Verification items for the finished model (mm, model axes). A direction names the side the tool comes from. Give positions to 0.01 mm unless a question says otherwise; leave off trailing zeros. Loops run counter-clockwise (first coordinate to the right, second up) from the corner with the lowest first, then second, coordinate; pieces in that order, holes last. Notation, with made-up numbers: M 39,36 L 43,36 A22 cw 43,60 Z; hole C 82.25,-23 d10. An arc over 180 degrees is marked long. Use CSV: the item, a comma, the result in double quotes.
from build123d import *

# Parameters (mm, degrees)
SKETCH1_R           = 1.905
BOSS_EXTRUDE1_DEPTH = 6.35
BOSS_EXTRUDE2_START = -6.35
BOSS_EXTRUDE2_DEPTH = 6.35
BOSS_EXTRUDE4_START = -6.35
SKETCH6_R           = 1.905
BOSS_EXTRUDE4_DEPTH = 6.35
SKETCH7_R           = 1.905
CUT_EXTRUDE3_DEPTH  = 15.340319034
SKETCH8_R           = 3.048
CUT_EXTRUDE4_DEPTH  = 2.54


with BuildPart() as part:
    # Sketch1 → Boss-Extrude1 (new body)
    with BuildSketch(Plane.YZ):
        with BuildLine():
            Line((-3.175, 0), (-3.175, -7.62))
            ThreePointArc((-3.175, -7.62), (0, -10.795), (3.175, -7.62))
            Line((3.175, -7.62), (3.175, 0))
            ThreePointArc((3.175, 0), (0, 3.175), (-3.175, 0))
        make_face()
        with Locations(Location((0, 0, 0), (0, 0, 270))):
            Circle(SKETCH1_R, mode=Mode.SUBTRACT)
    extrude(amount=BOSS_EXTRUDE1_DEPTH)

    # Sketch2 → Boss-Extrude2 (add)
    with BuildSketch(Plane.YZ.offset(6.35).offset(BOSS_EXTRUDE2_START)):
        with BuildLine():
            Line((4.445, -7.62), (4.445, 0))
            ThreePointArc((4.445, 0), (0, 4.445), (-4.445, 0))
            Line((-4.445, 0), (-4.445, -7.62))
            ThreePointArc((-4.445, -7.62), (0, -12.065), (4.445, -7.62))
        make_face()
        with BuildLine():
            ThreePointArc((3.175, 0), (0, 3.175), (-3.175, 0))
            Line((-3.175, 0), (-3.175, -7.62))
            ThreePointArc((-3.175, -7.62), (0, -10.795), (3.175, -7.62))
            Line((3.175, -7.62), (3.175, 0))
        make_face(mode=Mode.SUBTRACT)
    extrude(amount=BOSS_EXTRUDE2_DEPTH)

    # Sketch6 → Boss-Extrude4 (add)
    with BuildSketch(Plane.YZ.offset(6.35).offset(BOSS_EXTRUDE4_START)):
        Circle(SKETCH6_R)
    extrude(amount=BOSS_EXTRUDE4_DEPTH)

    # Sketch7 → Cut-Extrude3 (cut, through all)
    with BuildSketch(Plane(origin=(0, 0, 0), x_dir=(0, -1, 0), z_dir=(-1, 0, 0))):
        with Locations(Location((0, -1.27, 0), (0, 0, 90))):
            Circle(SKETCH7_R)
    extrude(amount=-CUT_EXTRUDE3_DEPTH, mode=Mode.SUBTRACT)

    # Sketch8 → Cut-Extrude4 (cut)
    with BuildSketch(Plane(origin=(0, 0, 0), x_dir=(0, -1, 0), z_dir=(-1, 0, 0))):
        with Locations(Location((0, -1.27, 0), (0, 0, 90))):
            Circle(SKETCH8_R)
    extrude(amount=-CUT_EXTRUDE4_DEPTH, mode=Mode.SUBTRACT)


solid = part.part
(1) Depth check by flat-ended pin: pin 1 Ø1 at (x, z) = (5, 1.5) entering from +Y. Enter the tip coordinate at first touch or a pass-through.
Calculated:
pin 1,"stops at y = 4.33"
(2) Section check B-B on z = 0.25. Record the cut outline in (x, y), plus the area to 3 significant figures.
Calculated:
outline,"M 0,-4.44 L 6.35,-4.44 L 6.35,-1.15 L 2.54,-1.15 L 2.54,-2.64 L 0,-2.64 Z; M 0,2.64 L 2.54,2.64 L 2.54,1.15 L 6.35,1.15 L 6.35,4.44 L 0,4.44 Z"
area,"34.2 mm²"
(3) Section check A-A on y = 0. Record the cut outline in (x, z) (3 decimals).
Calculated:
outline,"M 0,-12.065 L 6.35,-12.065 L 6.35,-3.175 L 2.54,-3.175 L 2.54,-4.318 L 0,-4.318 Z; M 0,1.778 L 2.54,1.778 L 2.54,0.635 L 6.35,0.635 L 6.35,4.445 L 0,4.445 Z"
(4) Tool access check on faces 1 (the cylindrical face through (1.252, 0.134, -4.315)), 2 (the flat face through (6.35, 0, -4)). Record the directions out of +Z, -Z, +X, -X, +Y, -Y that give a thin tool (end or side, any length) a straight path to the whole face; none if there is none.
Calculated:
face 1,"-X"
face 2,"+Z, -Z, +X, +Y, -Y"
(5) Mould release check, pull along Y, two halves, no side actions. Record for faces 3 (the cylindrical face through (4.42, 1.29, -2.67)), 4 (the flat face through (0, 0, -6)), 5 (the cylindrical face through (3.131, -0.098, -12.064)): released by +Y, released by -Y, zero draft, split by the parting line, or undercut.
Calculated:
face 3,"undercut"
face 4,"zero draft"
face 5,"split by the parting line"
(6) Section check D-D on y = 2.25. Record the cut outline in (x, z), plus the area to 3 significant figures.
Calculated:
outline,"M 0,-11.45 L 6.35,-11.45 L 6.35,3.83 L 0,3.83 L 0,0.79 L 2.54,0.79 L 2.54,-3.33 L 0,-3.33 Z"
area,"86.6 mm²"
(7) Section check C-C on x = 3.5. Record the cut outline in (y, z) (3 decimals).
Calculated:
outline,"M -4.445,-7.62 A4.445 ccw 4.445,-7.62 L 4.445,0 A4.445 ccw -4.445,0 Z; hole C 0,-1.27 d3.81"
(8) Scan lines: L1, parallel to Y at x = 1.35, z = -1.27 (3 decimals); L2, parallel to Y at x = 3.8, z = -1.27 (3 decimals); L3, parallel to Z at x = 4, y = -0.5. Record each from-to range of solid material in increasing order. Write a range as from..to.
Calculated:
L1,"y = -4.445..-3.048, 3.048..4.445"
L2,"y = -4.445..-1.905, 1.905..4.445"
L3,"z = -12.04..-3.11, 0.57..4.42"
